The model under review builds one solid part; all positions refer to its coordinate system, in mm. Face numbers are marked on the shaded views. A direction names the side the tool comes from. Coordinates: 2 decimals unless noted, no trailing zeros. Write each loop counter-clockwise with the first axis right and the second up, starting at its lowest first coordinate (ties: lowest second). Pieces come first, ordered by that corner, then holes. Notation, with made-up numbers: (44.5, 68) -> (49.5, 68) arc R28 ccw to (49.5, 88) -> close; hole circle Ø10 at (24, 22.5). An arc over 180 degrees is marked (long way). Put each result on its own line as item: value. Start each with the question number.
from build123d import *

# Parameters (mm, degrees)
SKETCH1_R                     = 95
BOSS_EXTRUDE1_DEPTH           = 70
SKETCH2_R                     = 80
CUT_EXTRUDE4_DEPTH            = 20
SKETCH5_R                     = 85
CUT_EXTRUDE5_DEPTH            = 10
RACCORDO1_R                   = 5
TAGLIO_ESTRUSIONE1_DEPTH      = 152.492574122
TAGLIO_ESTRUSIONE1_DEPTH_BACK = 152.492574122


with BuildPart() as part:
    # Sketch1 → Boss-Extrude1 (new, symmetric)
    with BuildSketch(Plane.XY):
        Circle(SKETCH1_R)
    extrude(amount=BOSS_EXTRUDE1_DEPTH, both=True)

    # Sketch2 → Cut-Extrude4 (cut)
    with BuildSketch(Plane(origin=(0, 0, -70), x_dir=(-1, 0, 0), z_dir=(0, 0, -1))):
        Circle(SKETCH2_R)
    extrude(amount=-CUT_EXTRUDE4_DEPTH, mode=Mode.SUBTRACT)

    # Sketch5 → Cut-Extrude5 (cut)
    with BuildSketch(Plane(origin=(0, 0, -50), x_dir=(-1, 0, 0), z_dir=(0, 0, -1))):
        Circle(SKETCH5_R)
    extrude(amount=-CUT_EXTRUDE5_DEPTH, mode=Mode.SUBTRACT)

    # Raccordo1
    raccordo1_edges = [part.edges().sort_by_distance(p)[0] for p in [
        (-95, 0, 70),
    ]]
    fillet(raccordo1_edges, radius=RACCORDO1_R)

    # Schizzo2 → Taglio-Estrusione1 (cut, two sides: drawn at the far end of the back side and taken through both)
    with BuildSketch(Plane(origin=(0, 0, 0), x_dir=(0, 0, -1), z_dir=(1, 0, 0)).offset(-TAGLIO_ESTRUSIONE1_DEPTH_BACK)):
        Polygon((24.150635095, 9.150635095), (-19.150635095, 34.150635095), (-44.150635095, -9.150635095), (-0.849364905, -34.150635095), align=None)
    extrude(amount=TAGLIO_ESTRUSIONE1_DEPTH + TAGLIO_ESTRUSIONE1_DEPTH_BACK, mode=Mode.SUBTRACT)


solid = part.part
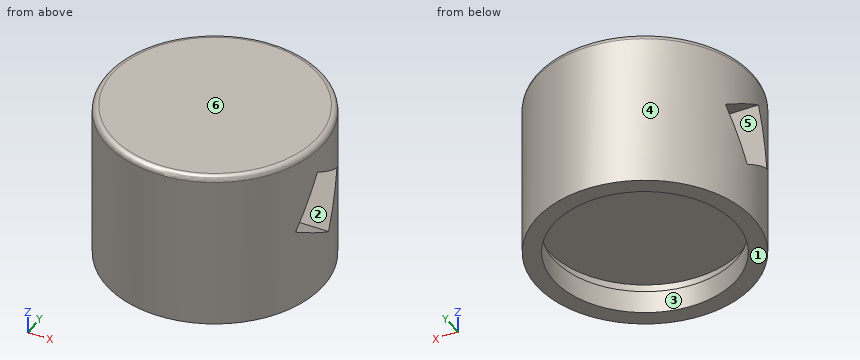
1. Wall thickness on line 1 (Y direction, x = 0, z = -54.75); line 2 (Y direction, x = 0, z = -44); line 3 (X direction, y = 1, z = 51.5): over which ranges is each line inside the solid? List them lowest first. Write a range as from..to.
2. Consider section A-A on x = 0. State the section outline as (y, z) points.
3. Consider section B-B on y = 0. State the section outline as (x, z) points, then the cut area to 3 significant figures.
4. Tool access review of the marked faces 5 and 6: name each direction out of +Z, -Z, +X, -X, +Y, -Y from which nothing blocks a thin tool from reaching the whole face with its end or side.
5. Insertion check: P1, Ø12, axis at y = -71, z = -13, coming from the +X side; P2, Ø1.5, axis at x = -24.5, z = 18.5, coming from the +Y side; P3, Ø1.5, axis at y = 28, z = -44.5, coming from the +X side. Each pin has a flat end and moves straight along its axis. Give the tip position at first contact, or say it passes through.
6. Consider section C-C on z = 56. State the section outline as (x, y) points.
7. The part is to be moulded in two halves that separate along Y. For the marked faces 1, 2, 3 and 4, say which applies: released by +Y, released by -Y, zero draft, split by the parting line, or undercut.
Output values:
1. line 1: y = -95..-80, 80..95
1. line 2: y = -95..-85, 85..95
1. line 3: x = -94.99..94.99
2. outline: (-95, -70) -> (-80, -70) -> (-80, -50) -> (-85, -50) -> (-85, -40) -> (85, -40) -> (85, -50) -> (80, -50) -> (80, -70) -> (95, -70) -> (95, 65) arc R5 ccw to (90, 70) -> (-90, 70) arc R5 ccw to (-95, 65) -> close; hole (-34.15, 0.85) -> (9.15, -24.15) -> (34.15, 19.15) -> (-9.15, 44.15) -> close
3. outline: (-95, -70) -> (-80, -70) -> (-80, -50) -> (-85, -50) -> (-85, -40) -> (85, -40) -> (85, -50) -> (80, -50) -> (80, -70) -> (95, -70) -> (95, -18.87) -> (-95, -18.87) -> close; (-95, 38.87) -> (95, 38.87) -> (95, 65) arc R5 ccw to (90, 70) -> (-90, 70) arc R5 ccw to (-95, 65) -> close
3. area: 10,700 mm^2
4. face 5: +X, -X
4. face 6: +Z, +X, -X, +Y, -Y
5. P1: stops at x = 69.28
5. P2: stops at y = 91.98
5. P3: stops at x = 91.01
6. outline: circle Ø190 at (0, 0)
7. face 1: zero draft
7. face 2: undercut
7. face 3: undercut
7. face 4: split by the parting line
